```python
from build123d import *

# Parameters (mm, degrees)
BOSS_EXTRUDE1_DEPTH = 65
SKETCH2_W           = 4
SKETCH2_H           = 4
SKETCH2_R           = 0.9
BOSS_EXTRUDE2_DEPTH = 5
CUT_EXTRUDE2_REACH  = 81.612
SKETCH3_W           = 16.5
SKETCH3_H           = 10.5
CUT_EXTRUDE3_REACH  = 82.864
CUT_EXTRUDE4_DEPTH  = 2
FILLET1_R           = 2.2
CUT_EXTRUDE5_REACH  = 81.687
SKETCH7_W           = 65
SKETCH7_H           = 12


with BuildPart() as part:
    # Sketch1 → Boss-Extrude1 (new body)
    with BuildSketch(Plane.XY):
        Polygon((0, 0), (33, 0), (33, 35), (30, 35), (30, 3), (0, 3), align=None)
    extrude(amount=BOSS_EXTRUDE1_DEPTH)

    # Sketch2 → Boss-Extrude2 (add)
    # profile 1 of 4: a face of its own
    with BuildSketch(Plane(origin=(0, 3, 0), x_dir=(1, 0, 0), z_dir=(0, 1, 0))):
        with Locations((25.25, -60.2)):
            Rectangle(SKETCH2_W, SKETCH2_H)
        with Locations(Location((25.25, -60.2, 0), (0, 0, 270))):
            Circle(SKETCH2_R, mode=Mode.SUBTRACT)
    # profile 2 of 4: a face of its own
    with BuildSketch(Plane(origin=(0, 3, 0), x_dir=(1, 0, 0), z_dir=(0, 1, 0))):
        with Locations((25.25, -4.8)):
            Rectangle(SKETCH2_W, SKETCH2_H)
        with Locations((25.25, -4.8)):
            Circle(SKETCH2_R, mode=Mode.SUBTRACT)
    # profile 3 of 4: a face of its own
    with BuildSketch(Plane(origin=(0, 3, 0), x_dir=(1, 0, 0), z_dir=(0, 1, 0))):
        with Locations((6, -5.1)):
            Rectangle(SKETCH2_W, SKETCH2_H)
        with Locations(Location((6, -5.1, 0), (0, 0, 270))):
            Circle(SKETCH2_R, mode=Mode.SUBTRACT)
    # profile 4 of 4: a face of its own
    with BuildSketch(Plane(origin=(0, 3, 0), x_dir=(1, 0, 0), z_dir=(0, 1, 0))):
        with Locations((5.2, -63)):
            Rectangle(SKETCH2_W, SKETCH2_H)
        with Locations(Location((5.2, -63, 0), (0, 0, 270))):
            Circle(SKETCH2_R, mode=Mode.SUBTRACT)
    extrude(amount=BOSS_EXTRUDE2_DEPTH)

    # Sketch3 → Cut-Extrude2 (cut, up to next)
    with BuildSketch(Plane(origin=(0, 3, 0), x_dir=(1, 0, 0), z_dir=(0, 1, 0)), mode=Mode.PRIVATE) as cut_extrude2_sk1:
        with Locations((21.75, -17.622736475)):
            Rectangle(SKETCH3_W, SKETCH3_H)
    cut_extrude2_tool1 = extrude(cut_extrude2_sk1.sketch, amount=-CUT_EXTRUDE2_REACH, mode=Mode.PRIVATE) & part.part
    add(cut_extrude2_tool1.solids().sort_by_distance((21.75, 3, 17.622736))[0], mode=Mode.SUBTRACT)

    # Sketch4 → Cut-Extrude3 (cut, up to next)
    with BuildSketch(Plane(origin=(33, 0, 0), x_dir=(0, 0, -1), z_dir=(1, 0, 0)), mode=Mode.PRIVATE) as cut_extrude3_sk1:
        with BuildLine():
            Line((-44.00188963, 16.3), (-50.99811037, 16.3))
            ThreePointArc((-50.99811037, 16.3), (-52.19811037, 17.5), (-50.99811037, 18.7))
            Line((-50.99811037, 18.7), (-44.00188963, 18.7))
            ThreePointArc((-44.00188963, 18.7), (-42.80188963, 17.5), (-44.00188963, 16.3))
        make_face()
    cut_extrude3_tool1 = extrude(cut_extrude3_sk1.sketch, amount=-CUT_EXTRUDE3_REACH, mode=Mode.PRIVATE) & part.part
    # Sketch4 → Cut-Extrude3 (cut, up to next)
    with BuildSketch(Plane(origin=(33, 0, 0), x_dir=(0, 0, -1), z_dir=(1, 0, 0)), mode=Mode.PRIVATE) as cut_extrude3_sk2:
        with BuildLine():
            Line((-20.99811037, 16.3), (-14.00188963, 16.3))
            ThreePointArc((-14.00188963, 16.3), (-12.80188963, 17.5), (-14.00188963, 18.7))
            Line((-14.00188963, 18.7), (-20.99811037, 18.7))
            ThreePointArc((-20.99811037, 18.7), (-22.19811037, 17.5), (-20.99811037, 16.3))
        make_face()
    cut_extrude3_tool2 = extrude(cut_extrude3_sk2.sketch, amount=-CUT_EXTRUDE3_REACH, mode=Mode.PRIVATE) & part.part
    add(cut_extrude3_tool1.solids().sort_by_distance((33, 17.5, 47.5))[0], mode=Mode.SUBTRACT)
    add(cut_extrude3_tool2.solids().sort_by_distance((33, 17.5, 17.5))[0], mode=Mode.SUBTRACT)

    # Sketch5 → Cut-Extrude4 (cut)
    with BuildSketch(Plane.ZY.offset(-30)):
        with BuildLine():
            Line((20.99811037, 14.95), (14.00188963, 14.95))
            ThreePointArc((14.00188963, 14.95), (11.45188963, 17.5), (14.00188963, 20.05))
            Line((14.00188963, 20.05), (20.99811037, 20.05))
            ThreePointArc((20.99811037, 20.05), (23.54811037, 17.5), (20.99811037, 14.95))
        make_face()
        with BuildLine():
            Line((44.00188963, 20.05), (50.99811037, 20.05))
            ThreePointArc((50.99811037, 20.05), (53.54811037, 17.5), (50.99811037, 14.95))
            Line((50.99811037, 14.95), (44.00188963, 14.95))
            ThreePointArc((44.00188963, 14.95), (41.45188963, 17.5), (44.00188963, 20.05))
        make_face()
    extrude(amount=-CUT_EXTRUDE4_DEPTH, mode=Mode.SUBTRACT)

    # Fillet1
    fillet1_edges = [part.edges().sort_by_distance(p)[0] for p in [
        (25.25, 3, 58.2),
        (27.25, 3, 60.2),
        (25.25, 3, 62.2),
        (23.25, 3, 60.2),
        (25.25, 3, 2.8),
        (23.25, 3, 4.8),
        (27.25, 3, 4.8),
        (25.25, 3, 6.8),
        (7.2, 3, 63),
        (5.2, 3, 61),
        (3.2, 3, 63),
        (8, 3, 5.1),
        (6, 3, 3.1),
        (6, 3, 7.1),
        (4, 3, 5.1),
    ]]
    fillet(fillet1_edges, radius=FILLET1_R)

    # Sketch7 → Cut-Extrude5 (cut, up to next)
    with BuildSketch(Plane.ZY.offset(-30), mode=Mode.PRIVATE) as cut_extrude5_sk1:
        with Locations((32.5, 29)):
            Rectangle(SKETCH7_W, SKETCH7_H)
    cut_extrude5_tool1 = extrude(cut_extrude5_sk1.sketch, amount=-CUT_EXTRUDE5_REACH, mode=Mode.PRIVATE) & part.part
    add(cut_extrude5_tool1.solids().sort_by_distance((30, 29, 32.5))[0], mode=Mode.SUBTRACT)


solid = part.part
```
Read the model definition and answer for the solid it produces. Units are mm, in the model's axes. A direction names the side the tool comes from. Give positions to 0.01 mm unless a question says otherwise; leave off trailing zeros. Loops run counter-clockwise (first coordinate to the right, second up) from the corner with the lowest first, then second, coordinate; pieces in that order, holes last.
Item 1: The part is cut by section B-B (x = 25.25). Write down the section's boundary in (y, z), and give its area (3 significant figures).
Item 2: The part is cut by section C-C (x = 17). Write down the section's boundary in (y, z).
Item 3: Find the intervals of material crossed by line 1 along X through (y, z) = (7, 63); line 2 along X through (y, z) = (5.9, 4.8); line 3 along X through (y, z) = (6.2, 5.1), in increasing order.
Item 4: The part is cut by section D-D (y = 9.5). Write down the section's boundary in (x, z).
Item 5: The part is cut by section A-A (z = 48). Write down the section's boundary in (x, y), and give its area (3 significant figures).
Item 6: The mould has two halves that part along X. Classify faces 5 (the flat face through (33, 11, 32)), 6 (the flat face through (20, 2, 65)), 7 (the flat face through (7.2, 7, 63)): released by +X, released by -X, zero draft, split by the parting line, or undercut.
Item 7: Each of these flat-tipped pins is pushed along its axis until it touches: pin 1 Ø1.2 at (x, z) = (6, 5.5) entering from +Y; pin 2 Ø1.4 at (x, z) = (6, 5.1) entering from +Y; pin 3 Ø2 at (x, y) = (25.5, 7) entering from -Z. Where does it stop, or does it pass through?
Item 8: For faces 1 (the cylindrical face through (6.059, 3.384, 2.142)), 2 (the flat face through (25, 7, 62.2)), 3 (the cylindrical face through (8.958, 3.384, 5.041)), 4 (the flat face through (6, 8, 4)), determine the directions among +Z, -Z, +X, -X, +Y, -Y from which every point of the face is accessible in a straight line to the end or side of a thin tool.
Taken from the geometry:
1. outline: (0, 0) - (3, 0) - (3, 0.6) arc R2.2 cw to (5.2, 2.8) - (8, 2.8) - (8, 3.9) - (3, 3.9) - (3, 5.7) - (8, 5.7) - (8, 6.8) - (5.2, 6.8) arc R2.2 cw to (3, 9) - (3, 12.37) - (0, 12.37) - close; (0, 22.87) - (3, 22.87) - (3, 56) arc R2.2 cw to (5.2, 58.2) - (8, 58.2) - (8, 59.3) - (3, 59.3) - (3, 61.1) - (8, 61.1) - (8, 62.2) - (5.2, 62.2) arc R2.2 cw to (3, 64.4) - (3, 65) - (0, 65) - close
1. area: 190 mm2
2. outline: (0, 0) - (3, 0) - (3, 12.37) - (0, 12.37) - close; (0, 22.87) - (3, 22.87) - (3, 65) - (0, 65) - close
3. line 1: x = 3.2 to 4.3, 6.1 to 7.2, 30 to 33
3. line 2: x = 4 to 5.15, 6.85 to 8, 23.25 to 24.35, 26.15 to 27.25, 30 to 33
3. line 3: x = 4 to 5.1, 6.9 to 8, 23.25 to 24.4, 26.1 to 27.25, 30 to 33
4. outline: (30, 0) - (33, 0) - (33, 65) - (30, 65) - close
5. outline: (0, 0) - (33, 0) - (33, 16.3) - (32, 16.3) - (32, 14.95) - (30, 14.95) - (30, 3) - (0, 3) - close; (30, 20.05) - (32, 20.05) - (32, 18.7) - (33, 18.7) - (33, 23) - (30, 23) - close
5. area: 146 mm2
6. face 5: released by +X
6. face 6: zero draft
6. face 7: undercut
7. pin 1: stops at y = 8
7. pin 2: stops at y = 3
7. pin 3: stops at z = 2.8
8. face 1: -Z, -X, +Y
8. face 2: +Z, +Y
8. face 3: +Z, -Z, +Y
8. face 4: +Z, -Z, -X, +Y
